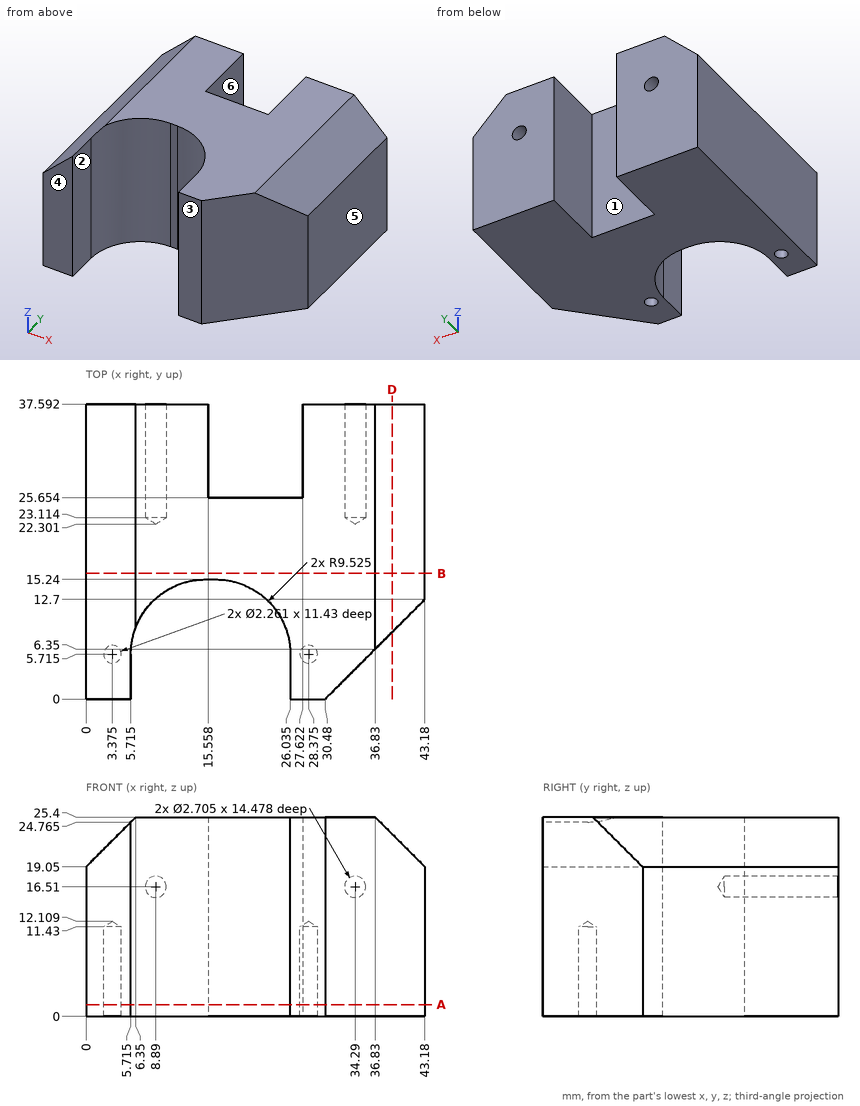
For this review, use the dimensioned drawing (mm, ordinates from the lowest corner) and the shaded views. A direction names the side the tool comes from. Round coordinates to 2 decimals unless told otherwise and drop trailing zeros. Loops run counter-clockwise (first coordinate to the right, second up) from the corner with the lowest first, then second, coordinate; pieces in that order, holes last. Notation, with made-up numbers: M -16.5,-38 L 26.5,-38 A20 ccw 26.5,-20 Z; hole C 77,63.5 d11. An arc over 180 degrees is marked long. Answer as a JSON object with one key per item and string values.
(1) To check wall thickness, follow line 1 along X through (y, z) = (33, 16.51); line 2 along Z through (x, y) = (34.29, 33); line 3 along Y through (x, z) = (28.5, 9). State the ranges of each line that lie inside material, in increasing order.
Resolved:
{"line 1": "0 to 7.54, 10.24 to 15.56, 27.62 to 32.94, 35.64 to 43.18", "line 2": "0 to 15.16, 17.86 to 25.4", "line 3": "0 to 4.59, 6.84 to 37.59"}
(2) Take a section at D-D on x = 39. Give the boundary of the cut face in (y, z), and give its area (3 significant figures).
Resolved:
{"outline": "M 8.52,0 L 37.59,0 L 37.59,23.23 L 8.52,23.23 Z", "area": "675 mm²"}
(3) Take a section at A-A on z = 1.5. Count the separate pieces of the cut face and the enclosed holes in it, and give its area (3 significant figures).
Resolved:
{"separate pieces": "1", "enclosed holes": "2", "area": "1,120 mm²"}
(4) Clearance check with flat-ended pins moving along their axes: P1, Ø1.4, axis at x = 3.375, y = 5.715, coming from the +Z side (1 decimal); P2, Ø4.5, axis at y = 2, z = 13, coming from the +X side; P3, Ø1.5, axis at y = 6, z = 22, coming from the -X side. State where each tip first meets the part, or that it passes through.
Resolved:
{"P1": "z = 23.1", "P2": "x = 34.73", "P3": "x = 2.2"}
(5) Tool access review of the marked faces 1, 2 and 3: name each direction out of +Z, -Z, +X, -X, +Y, -Y from which nothing blocks a thin tool from reaching the whole face with its end or side.
Resolved:
{"face 1": "+Z, -Z, +Y", "face 2": "+Z, -Z, -Y", "face 3": "+Z, -Z, +X, -X, -Y"}
(6) Draft analysis for pull direction X (two halves, no side actions). For the marked faces 4, 5 and 6, state which applies: released by +X, released by -X, zero draft, split by the parting line, or undercut.
Resolved:
{"face 4": "zero draft", "face 5": "released by +X", "face 6": "undercut"}
(7) Take a section at B-B on y = 16. Give the boundary of the cut face in (x, z).
Resolved:
{"outline": "M 0,0 L 43.18,0 L 43.18,19.05 L 36.83,25.4 L 6.35,25.4 L 0,19.05 Z"}
